Autodesk Inventor part; units mm, degrees
ref_plane "bolt_XY" through (0, 0, 0) normal (1, 0, 0) x (0, 0, -1)
ref_plane "bolt_YZ" through (0, 0, 0) normal (0, 0, -1) x (0, 1, 0)
ref_plane "bolt_ZX" through (0, 0, 0) normal (0, 1, 0) x (1, 0, 0)
sketch "Sketch_1" plane through (0, 0, 0) normal (0, 0, 1) x (1, 0, 0)
  line L0 (10, 0) -> (-2, 0)
  line L1 (-2, 0) -> (-2, 2.75)
  line L2 (-2, 2.75) -> (0, 2.75)
  line L3 (0, 2.75) -> (0, 1.6)
  arc A0 (0, 1.6) -> (0.1, 1.5) centre (0.1, 1.6) ccw
  line L4 (0.1, 1.5) -> (9.6935, 1.5)
  line L5 (9.6935, 1.5) -> (10, 1.1935)
  line L6 (10, 1.1935) -> (10, 0)
  line L7 (10, 0) -> (-2, 0)
revolve "Revolution1" add sketch "Sketch_1" angle 360 about axis through (10, 0, 0) along (1, 0, 0)
thread "Thread1"
sketch "Sketch2" plane through (-2, 0, 0) normal (-1, 0, 0) x (0, 0, 1)
  point P0 (0, 0)
hole "Hole1" at (-2, 0, 0) direction (1, 0, 0) diameter 2 depth 1.5 tip angle 140
sketch "Sketch_3" plane through (-2, 0, 0) normal (1, 0, 0) x (0, 0, -1)
  line L0 (-1, 0.5774) -> (-1, -0.5774)
  line L1 (-1, -0.5774) -> (0, -1.1547)
  line L2 (0, -1.1547) -> (1, -0.5774)
  line L3 (1, -0.5774) -> (1, 0.5774)
  line L4 (1, 0.5774) -> (0, 1.1547)
  line L5 (0, 1.1547) -> (-1, 0.5774)
extrude "Extrusion1" cut sketch "Sketch_3" along normal blind 1.5
ref_plane "bolt_XY" through (0, 0, 0) normal (1, 0, 0) x (0, 0, -1)
ref_plane "bolt_YZ" through (0, 0, 0) normal (0, 0, -1) x (0, 1, 0)
ref_plane "bolt_ZX" through (0, 0, 0) normal (0, 1, 0) x (1, 0, 0)
ref_plane "bolt_to_nut_XY" through (10, 0, 0) normal (1, 0, 0) x (0, 0, -1)
ref_plane "bolt_to_nut_YZ" through (10, 0, 0) normal (0, 0, -1) x (0, 1, 0)
ref_plane "bolt_to_nut_ZX" through (10, 0, 0) normal (0, 1, 0) x (1, 0, 0)
properties part number "CBS3-10"
Model file for the job. Use its own axes, mm. A direction names the side the tool comes from. Coordinates: 2 decimals unless noted, no trailing zeros. Order: outer loops, then holes, each group sorted by start corner. A loop starts at its lowest first (then second) coordinate and runs counter-clockwise, first axis right, second up. Notation, with made-up numbers: (23.5, 9) - (58.5, 9) arc R13 cw to (58.5, 20) - close; hole circle Ø11 at (-29.5, 1). An arc over 180 degrees is marked (long way). Return JSON: item names as keys, results as strings. Group by question number.
1) Mould opens along Y. For faces 3 (the conical face through (-0.16, -0.06, -0.01)), 4 (the flat face through (0, 2, 0)), 5 (the cylindrical face through (4.96, -1.5, 0.07)) say: released by +Y, released by -Y, zero draft, split by the parting line, or undercut.
2) Probe line 1 (X direction, y = -2, z = 0.05); line 2 (Z direction, x = 5.25, y = 0); line 3 (Y direction, x = -1, z = -0.3). List the from-to ranges inside material, lowest first. Write a range as from..to.
3) Saw through at A-A, the plane x = -0.75. Write the cut outline in (y, z), plus the area to 3 significant figures.
4) Saw through at B-B, the plane x = 6.5. Write the cut outline in (y, z).
5) Saw through at C-C, the plane z = -2.05. Write the cut outline in (x, y), plus the area to 3 significant figures.
6) Saw through at D-D, the plane y = 1.9. Write the cut outline in (x, z), plus the area to 3 significant figures.
7) Flat gauge pin, fed straight in: P1, Ø1, axis at x = 1.5, z = 1.5, coming from the +Y side. Where does the tip first touch, or does it go through?
8) Tool access for faces 1 (the flat face through (-1, 0, -1)), 2 (the flat face through (-2, 0, -1.2)): list every direction of +Z, -Z, +X, -X, +Y, -Y with a clear straight run to the whole face (end or side of a thin tool).
Values found:
{
 "1": {"face 3": "undercut", "face 4": "zero draft", "face 5": "split by the parting line"},
 "2": {"line 1": "x = -2..0", "line 2": "z = -1.5..1.5", "line 3": "y = -2.73..-0.98, 0.98..2.73"},
 "3": {"outline": "circle Ø5.5 at (0, 0); hole (-1.15, 0) - (-0.58, -1) - (0.58, -1) - (1.15, 0) - (0.58, 1) - (-0.58, 1) - close", "area": "20.3 mm²"},
 "4": {"outline": "circle Ø3 at (0, 0)"},
 "5": {"outline": "(-2, -1.83) - (0, -1.83) - (0, 1.83) - (-2, 1.83) - close", "area": "7.33 mm²"},
 "6": {"outline": "(-2, -1.99) - (0, -1.99) - (0, 1.99) - (-2, 1.99) - close", "area": "7.95 mm²"},
 "7": {"P1": "stops at y = 1.12"},
 "8": {"face 1": "-X", "face 2": "+Z, -Z, -X, +Y, -Y"}
}
